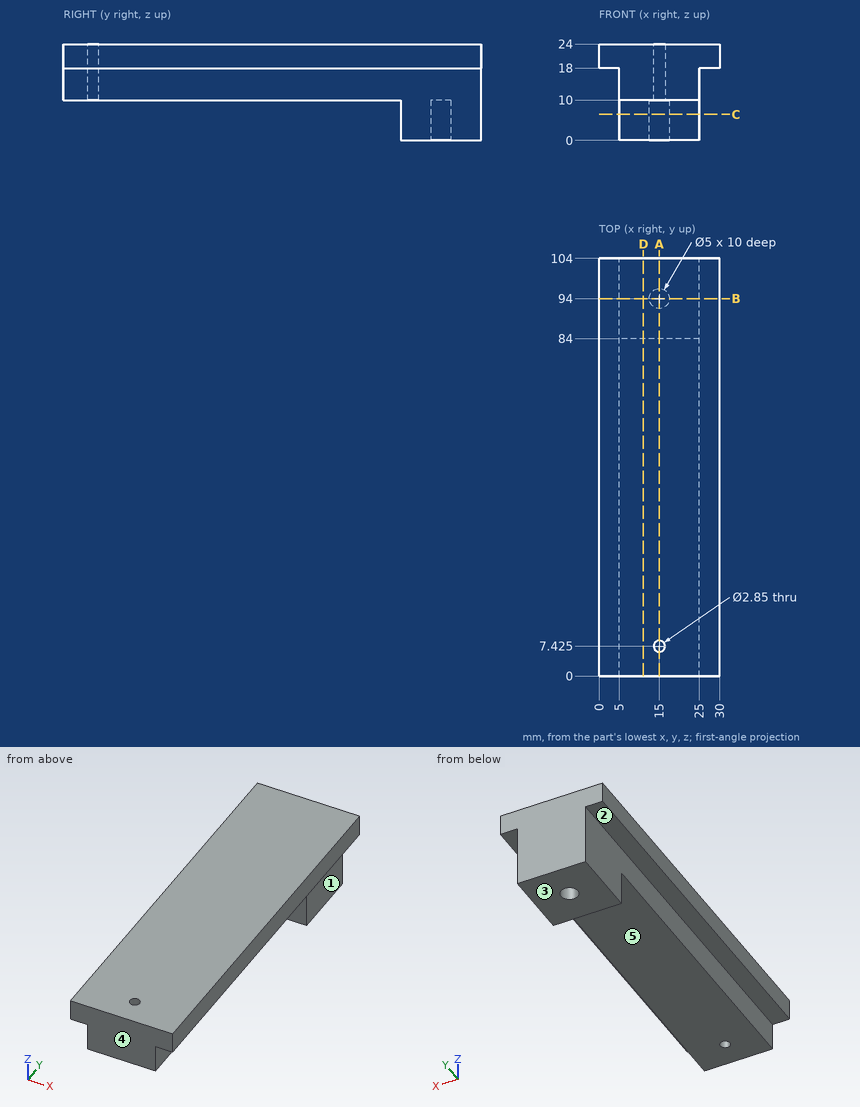
Print and shaded views of the part. All mm, measured from the part's lowest x, y and z. A direction names the side the tool comes from. Coordinates: 2 decimals unless noted, no trailing zeros. Loops run counter-clockwise (first coordinate to the right, second up) from the corner with the lowest first, then second, coordinate; pieces in that order, holes last. Notation, with made-up numbers: (12.25, 49.5) -> (62.25, 49.5) arc R19 cw to (62.25, 82.5) -> close; hole circle Ø1 at (13, -19.5). An arc over 180 degrees is marked (long way). Use a Markdown table: item, result. Add a question column.
Item 1: Probe probe 1 along Y at (x, z) = (15, 5.25); probe 2 along Y at (x, z) = (15, 15.5); probe 3 along Z at (x, y) = (2.5, 51.5). List the from-to ranges inside material, lowest first.
Item 2: Which spindle directions (+Z, -Z, +X, -X, +Y, -Y) get a long thin tool onto all of the face, cutting with end or side? Do the marked faces 1, 2, 3, 4 and 5. Say none if no direction does.
Item 3: Band-saw the part on A-A on x = 15. Write the cut outline in (y, z).
Item 4: Flat gauge pins, fed straight in: P1, Ø5.5, axis at y = 51.5, z = 12.5, coming from the -X side; P2, Ø1.5, axis at y = 34.5, z = 13, coming from the +X side; P3, Ø2, axis at x = 3.5, y = 78, coming from the -Z side. Where does each tip first touch, or does it go through?
Item 5: Band-saw the part on B-B on y = 94. Write the cut outline in (x, z).
Item 6: Band-saw the part on C-C on z = 6.5. Write the cut outline in (x, y), plus the area to 3 significant figures.
Item 7: Band-saw the part on D-D on x = 11. Write the cut outline in (y, z), plus the area to 3 significant figures.
Geometry says:
| question | item | result |
|---|---|---|
| 1 | probe 1 | 84 to 91.5, 96.5 to 104 |
| 1 | probe 2 | 0 to 6, 8.85 to 104 |
| 1 | probe 3 | 18 to 24 |
| 2 | face 1 | -Z, +X, +Y, -Y |
| 2 | face 2 | -Z, -X, +Y, -Y |
| 2 | face 3 | -Z, +X, -X, +Y, -Y |
| 2 | face 4 | +Z, -Z, +X, -X, -Y |
| 2 | face 5 | -Z, +X, -X, -Y |
| 3 | outline | (0, 10) -> (6, 10) -> (6, 24) -> (0, 24) -> close; (8.85, 10) -> (84, 10) -> (84, 0) -> (91.5, 0) -> (91.5, 10) -> (96.5, 10) -> (96.5, 0) -> (104, 0) -> (104, 24) -> (8.85, 24) -> close |
| 4 | P1 | x = 5 |
| 4 | P2 | x = 25 |
| 4 | P3 | z = 18 |
| 5 | outline | (0, 18) -> (5, 18) -> (5, 0) -> (12.5, 0) -> (12.5, 10) -> (17.5, 10) -> (17.5, 0) -> (25, 0) -> (25, 18) -> (30, 18) -> (30, 24) -> (0, 24) -> close |
| 6 | outline | (5, 84) -> (25, 84) -> (25, 104) -> (5, 104) -> close; hole circle Ø5 at (15, 94) |
| 6 | area | 380 mm² |
| 7 | outline | (0, 10) -> (84, 10) -> (84, 0) -> (104, 0) -> (104, 24) -> (0, 24) -> close |
| 7 | area | 1,660 mm² |
